Read the model definition and answer for the solid it produces. Units are mm, in the model's axes. A direction names the side the tool comes from. Give positions to 0.01 mm unless a question says otherwise; leave off trailing zeros. Order: outer loops, then holes, each group sorted by start corner. A loop starts at its lowest first (then second) coordinate and runs counter-clockwise, first axis right, second up. Notation, with made-up numbers: (-3, 56.5) -> (54, 56.5) arc R28 cw to (54, 81.5) -> close; hole circle Ø7 at (-1, 79.25). An arc over 180 degrees is marked (long way). Use one line per item in the form item = value.
```python
from build123d import *

# Parameters (mm, degrees)
SKETCH1_R           = 4.25
BOSS_EXTRUDE1_DEPTH = 12.7
SKETCH3_R           = 4.25
BOSS_EXTRUDE3_DEPTH = 12.7
SKETCH4_R           = 4.25
BOSS_EXTRUDE4_DEPTH = 19.05
SKETCH5_R           = 3.2385
CUT_EXTRUDE1_DEPTH  = 140.157754455


with BuildPart() as part:
    # Sketch1 → Boss-Extrude1 (new body)
    with BuildSketch(Plane.XY):
        with BuildLine():
            Line((93.98, -12.7), (-93.98, -12.7))
            ThreePointArc((-93.98, -12.7), (-96.674076836, -11.584076836), (-97.79, -8.89))
            Line((-97.79, -8.89), (-97.79, 8.89))
            ThreePointArc((-97.79, 8.89), (-96.674076836, 11.584076836), (-93.98, 12.7))
            Line((-93.98, 12.7), (93.98, 12.7))
            ThreePointArc((93.98, 12.7), (96.674076836, 11.584076836), (97.79, 8.89))
            Line((97.79, 8.89), (97.79, -8.89))
            ThreePointArc((97.79, -8.89), (96.674076836, -11.584076836), (93.98, -12.7))
        make_face()
        with Locations((-88.9, 0)):
            Circle(SKETCH1_R, mode=Mode.SUBTRACT)
        with Locations((88.9, 0)):
            Circle(SKETCH1_R, mode=Mode.SUBTRACT)
    extrude(amount=BOSS_EXTRUDE1_DEPTH)

    # Sketch3 → Boss-Extrude3 (add, through all)
    with BuildSketch(Plane.XY.offset(12.7)):
        with BuildLine():
            Line((-6.335384206, -97.155), (6.335384206, -97.155))
            ThreePointArc((6.335384206, -97.155), (9.927486654, -95.667102448), (11.415384206, -92.075))
            Line((11.415384206, -92.075), (11.415384206, 92.075))
            ThreePointArc((11.415384206, 92.075), (9.927486654, 95.667102448), (6.335384206, 97.155))
            Line((6.335384206, 97.155), (-6.335384206, 97.155))
            ThreePointArc((-6.335384206, 97.155), (-9.927486654, 95.667102448), (-11.415384206, 92.075))
            Line((-11.415384206, 92.075), (-11.415384206, -92.075))
            ThreePointArc((-11.415384206, -92.075), (-9.927486654, -95.667102448), (-6.335384206, -97.155))
        make_face()
        with Locations((0, 88.9)):
            Circle(SKETCH3_R, mode=Mode.SUBTRACT)
        with Locations((0, -88.9)):
            Circle(SKETCH3_R, mode=Mode.SUBTRACT)
    extrude(amount=-BOSS_EXTRUDE3_DEPTH)

    # Sketch4 → Boss-Extrude4 (add)
    # profile 1 of 4: a face of its own
    with BuildSketch(Plane.XY.offset(12.7)):
        with BuildLine():
            Line((-81.28, 12.7), (-93.98, 12.7))
            ThreePointArc((-93.98, 12.7), (-96.674076836, 11.584076836), (-97.79, 8.89))
            Line((-97.79, 8.89), (-97.79, -8.89))
            ThreePointArc((-97.79, -8.89), (-96.674076836, -11.584076836), (-93.98, -12.7))
            Line((-93.98, -12.7), (-81.28, -12.7))
            Line((-81.28, -12.7), (-81.28, 12.7))
        make_face()
        with Locations((-88.9, 0)):
            Circle(SKETCH4_R, mode=Mode.SUBTRACT)
    # profile 2 of 4: a face of its own
    with BuildSketch(Plane.XY.offset(12.7)):
        with BuildLine():
            Line((-11.415384206, 92.075), (-11.415384206, 80.645))
            Line((-11.415384206, 80.645), (11.415384206, 80.645))
            Line((11.415384206, 80.645), (11.415384206, 92.075))
            ThreePointArc((11.415384206, 92.075), (9.927486654, 95.667102448), (6.335384206, 97.155))
            Line((6.335384206, 97.155), (-6.335384206, 97.155))
            ThreePointArc((-6.335384206, 97.155), (-9.927486654, 95.667102448), (-11.415384206, 92.075))
        make_face()
        with Locations((0, 88.9)):
            Circle(SKETCH4_R, mode=Mode.SUBTRACT)
    # profile 3 of 4: a face of its own
    with BuildSketch(Plane.XY.offset(12.7)):
        with BuildLine():
            Line((93.98, 12.7), (81.28, 12.7))
            Line((81.28, 12.7), (81.28, -12.7))
            Line((81.28, -12.7), (93.98, -12.7))
            ThreePointArc((93.98, -12.7), (96.674076836, -11.584076836), (97.79, -8.89))
            Line((97.79, -8.89), (97.79, 8.89))
            ThreePointArc((97.79, 8.89), (96.674076836, 11.584076836), (93.98, 12.7))
        make_face()
        with Locations((88.9, 0)):
            Circle(SKETCH4_R, mode=Mode.SUBTRACT)
    # profile 4 of 4: a face of its own
    with BuildSketch(Plane.XY.offset(12.7)):
        with BuildLine():
            Line((11.415384206, -80.645), (-11.415384206, -80.645))
            Line((-11.415384206, -80.645), (-11.415384206, -92.075))
            ThreePointArc((-11.415384206, -92.075), (-9.927486654, -95.667102448), (-6.335384206, -97.155))
            Line((-6.335384206, -97.155), (6.335384206, -97.155))
            ThreePointArc((6.335384206, -97.155), (9.927486654, -95.667102448), (11.415384206, -92.075))
            Line((11.415384206, -92.075), (11.415384206, -80.645))
        make_face()
        with Locations((0, -88.9)):
            Circle(SKETCH4_R, mode=Mode.SUBTRACT)
    extrude(amount=BOSS_EXTRUDE4_DEPTH)

    # Sketch5 → Cut-Extrude1 (cut, through all)
    with BuildSketch(Plane.XY.offset(12.7)):
        with Locations((0, 63.5)):
            Circle(SKETCH5_R)
        with Locations((63.5, 0)):
            Circle(SKETCH5_R)
        with Locations((0, -63.5)):
            Circle(SKETCH5_R)
        with Locations((-63.5, 0)):
            Circle(SKETCH5_R)
    extrude(amount=-CUT_EXTRUDE1_DEPTH, mode=Mode.SUBTRACT)


solid = part.part
```
Item 1: The part is cut by section B-B on x = -63.5. Give the vertices of the cut face in (y, z).
Checks:
outline = (-12.7, 0) -> (-3.24, 0) -> (-3.24, 12.7) -> (-12.7, 12.7) -> close; (3.24, 0) -> (12.7, 0) -> (12.7, 12.7) -> (3.24, 12.7) -> close
Item 2: Given pin 1 Ø3 at (x, z) = (62, 10) entering from +Y; pin 2 Ø1 at (x, z) = (54.5, 7) entering from -Y; pin 3 Ø4 at (y, z) = (-70, 14) entering from +X, each flat-ended and moving along its own axis, determine where each tip first touches the part or whether it passes through.
Checks:
pin_1 = 12.7
pin_2 = -12.7
pin_3 = 11.42
Item 3: Straight lines are drawn through the part: L1, parallel to Z at x = 4.5, y = 65; L2, parallel to X at y = 42, z = 10; L3, parallel to X at y = -86.5, z = 17.5. For each, find the intervals that lie inside material, in ascending order. Write a range as from..to.
Checks:
L1 = 0..12.7
L2 = -11.42..11.42
L3 = -11.42..-3.51, 3.51..11.42
Item 4: The part is cut by section C-C on y = 0. Give the vertices of the cut face in (x, z), and give its area (3 significant figures).
Checks:
outline = (-97.79, 0) -> (-93.15, 0) -> (-93.15, 31.75) -> (-97.79, 31.75) -> close; (-84.65, 0) -> (-66.74, 0) -> (-66.74, 12.7) -> (-81.28, 12.7) -> (-81.28, 31.75) -> (-84.65, 31.75) -> close; (-60.26, 0) -> (60.26, 0) -> (60.26, 12.7) -> (-60.26, 12.7) -> close; (66.74, 0) -> (84.65, 0) -> (84.65, 31.75) -> (81.28, 31.75) -> (81.28, 12.7) -> (66.74, 12.7) -> close; (93.15, 0) -> (97.79, 0) -> (97.79, 31.75) -> (93.15, 31.75) -> close
area = 2,410 mm²
Item 5: Which of the six approach directions +Z, -Z, +X, -X, +Y, -Y give full straight-line access (tool end or side, diameter ignored) to faces 5 (the flat face through (52, 12.7, 9)), 6 (the flat face through (53, -12.7, 9)), 7 (the flat face through (-81.28, 0, 22))?
Checks:
face_5 = +Z, -Z, +X, +Y
face_6 = +Z, -Z, +X, -Y
face_7 = +Z, +Y, -Y
Item 6: The part is cut by section D-D on y = 88.9. Give the vertices of the cut face in (x, z), and give its area (3 significant figures).
Checks:
outline = (-11.42, 0) -> (-4.25, 0) -> (-4.25, 31.75) -> (-11.42, 31.75) -> close; (4.25, 0) -> (11.42, 0) -> (11.42, 31.75) -> (4.25, 31.75) -> close
area = 455 mm²
Item 7: The part is cut by section A-A on z = 22.5. Give the vertices of the cut face in (x, y) (3 decimals), and give its area (3 significant figures).
Checks:
outline = (-97.79, -8.89) arc R3.81 ccw to (-93.98, -12.7) -> (-81.28, -12.7) -> (-81.28, 12.7) -> (-93.98, 12.7) arc R3.81 ccw to (-97.79, 8.89) -> close; (-11.415, -92.075) arc R5.08 ccw to (-6.335, -97.155) -> (6.335, -97.155) arc R5.08 ccw to (11.415, -92.075) -> (11.415, -80.645) -> (-11.415, -80.645) -> close; (-11.415, 80.645) -> (11.415, 80.645) -> (11.415, 92.075) arc R5.08 ccw to (6.335, 97.155) -> (-6.335, 97.155) arc R5.08 ccw to (-11.415, 92.075) -> close; (81.28, -12.7) -> (93.98, -12.7) arc R3.81 ccw to (97.79, -8.89) -> (97.79, 8.89) arc R3.81 ccw to (93.98, 12.7) -> (81.28, 12.7) -> close; hole circle Ø8.5 at (-88.9, 0); hole circle Ø8.5 at (0, -88.9); hole circle Ø8.5 at (0, 88.9); hole circle Ø8.5 at (88.9, 0)
area = 1,330 mm²
Item 8: Determine the mould class of faces 1 (the flat face through (-11.415, -52, 9)), 2 (the flat face through (-53, -12.7, 9)), 3 (the cylindrical face through (66.49, -1.24, 6.44)), 4 (the cylindrical face through (9.888, -95.706, 16.097)) for opening direction X: +X half, -X half, draft (parallel to the pull), parting line (faces both ways), or undercut.
Checks:
face_1 = -X half
face_2 = draft
face_3 = undercut
face_4 = +X half
